Source: three-view drawing plus pictorial views. Frame: mm from the lowest corner of the part. Give positions to 0.01 mm unless a question says otherwise; leave off trailing zeros. Order: outer loops, then holes, each group sorted by start corner. A loop starts at its lowest first (then second) coordinate and runs counter-clockwise, first axis right, second up.
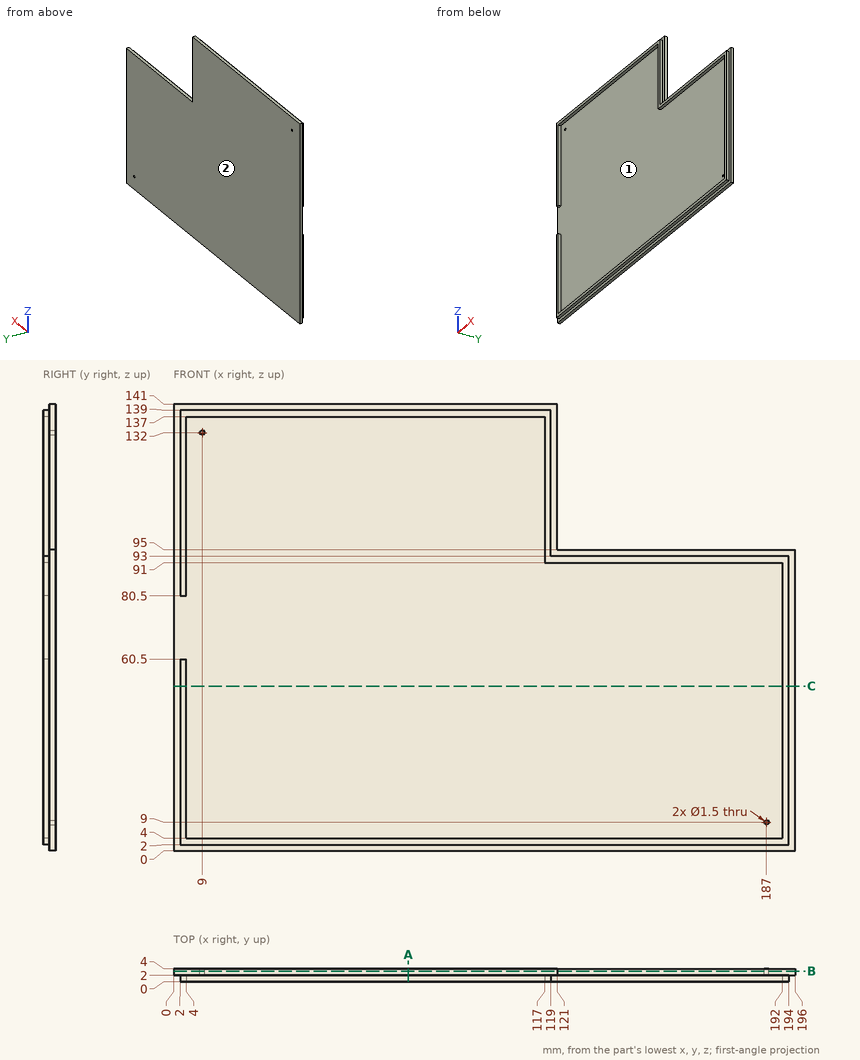
(1) Section C-C, the plane z = 52. Return loops of the section in (x, y).
(2) Section B-B, the plane y = 3.3. Return loops of the section in (x, z), plus the area to 3 significant figures.
(3) Section A-A, the plane x = 74. Return loops of the section in (y, z).
(4) Line query: line 1 along Z through (x, y) = (155, 0.2); line 2 along Z through (x, y) = (187, 3.55); line 3 along X through (y, z) = (3.6, 132). Output: solid intervals per line, ascending.
(5) Draft query along Z for the marked faces 1 and 2. Return one class per face: +Z half, -Z half, draft (parallel to the pull), parting line (faces both ways), or undercut.
(6) Pin query (flat end, axial travel): pin 1 Ø0.6 at (y, z) = (1, 109.5) entering from +X; pin 2 Ø1.6 at (x, y) = (69, 1) entering from -Z; pin 3 Ø2 at (y, z) = (0.5, 32.5) entering from -X. Return the tip coordinate at first contact, or that it passes through.
Checks:
1. outline: (0, 2) - (2, 2) - (2, 0) - (4, 0) - (4, 2) - (192, 2) - (192, 0) - (194, 0) - (194, 2) - (196, 2) - (196, 4) - (0, 4) - close
2. outline: (0, 0) - (196, 0) - (196, 95) - (121, 95) - (121, 141) - (0, 141) - close; hole circle Ø1.5 at (9, 132); hole circle Ø1.5 at (187, 9)
2. area: 24,200 mm2
3. outline: (0, 2) - (2, 2) - (2, 0) - (4, 0) - (4, 141) - (2, 141) - (2, 139) - (0, 139) - (0, 137) - (2, 137) - (2, 4) - (0, 4) - close
4. line 1: z = 2 to 4, 91 to 93
4. line 2: z = 0 to 8.25, 9.75 to 95
4. line 3: x = 0 to 8.25, 9.75 to 121
5. face 1: undercut
5. face 2: draft
6. pin 1: stops at x = 119
6. pin 2: stops at z = 2
6. pin 3: stops at x = 2
